The listing builds one solid part. Answer for the finished solid, in the listing's coordinates (mm). Face numbers are marked on the shaded views. A direction names the side the tool comes from. Give positions to 0.01 mm unless a question says otherwise; leave off trailing zeros. Order: outer loops, then holes, each group sorted by start corner. A loop starts at its lowest first (then second) coordinate and runs counter-clockwise, first axis right, second up. Notation, with made-up numbers: (-22.75, 14.25) -> (18.25, 14.25) arc R29 cw to (18.25, 49.25) -> close; hole circle Ø5 at (-2.5, 35.25). An arc over 180 degrees is marked (long way). Answer as a JSON object with one key per item and string values. Group by question number.
Autodesk Inventor part; units mm, degrees
ref_plane "YZ Plane" through (0, 0, 0) normal (1, 0, 0) x (0, 1, 0)
ref_plane "XZ Plane" through (0, 0, 0) normal (0, 1, 0) x (-1, 0, 0)
ref_plane "XY Plane" through (0, 0, 0) normal (0, 0, 1) x (1, 0, 0)
sketch "Sketch1" plane through (0, 0, 0) normal (0, 1, 0) x (-1, 0, 0)
  line L0 (22.5, 35) -> (-22.5, 35)
  line L1 (-22.5, 35) -> (-22.5, -35)
  line L2 (-22.5, -35) -> (22.5, -35)
  line L3 (22.5, -35) -> (22.5, 35)
  line L4 (22.5, 35) -> (-22.5, -35) construction
  line L5 (-22.5, 35) -> (22.5, -35) construction
  line L6 (0, 0) -> (0, -35) construction
  circle A0 centre (0, -25) radius 2.5
  circle A1 centre (0, -25) radius 4.5 construction
  line L7 (0, -25) -> (-4.5, -25) construction
  circle A2 centre (-4.5, -25) radius 0.625
  circle A3 centre (-6.5, -25) radius 0.625
  circle A4 centre (-8.5, -25) radius 0.625
  circle A5 centre (-10.5, -25) radius 0.625
  circle A6 centre (-12.5, -25) radius 0.625
  circle A7 centre (-14.5, -25) radius 0.625
  circle A8 centre (4.5, -25) radius 0.625
  circle A9 centre (6.5, -25) radius 0.625
  circle A10 centre (8.5, -25) radius 0.625
  circle A11 centre (10.5, -25) radius 0.625
  circle A12 centre (12.5, -25) radius 0.625
  circle A13 centre (14.5, -25) radius 0.625
  dimension "d3" = 9
  dimension "d0" = 45
  dimension "d1" = 70
  dimension "d2" = 5
  dimension "d4" = 1.25
  dimension "d7" = 2
  dimension "d14" = 360
  dimension "d16" = 10
extrude "Extrusion1" add sketch "Sketch1" along normal blind 3.175
fillet "Fillet1" radius 3.175 4 edges at (22.5, 1.5875, -35) (-22.5, 1.5875, -35) (-22.5, 1.5875, 35) (22.5, 1.5875, 35)
sketch "Sketch2" plane through (0, 3.175, 0) normal (0, 1, 0) x (1, 0, 0)
  line L0 (-22.5, 31.825) -> (-22.5, -31.825)
  line L1 (-22.5, 15) -> (22.5, 15)
  line L2 (22.5, -31.825) -> (22.5, 31.825)
  line L3 (19.325, 35) -> (-19.325, 35)
  point P0 (0, 0)
  dimension "d20" = 20
bend part "Bend Part1" radius 3 angle 90 line through (-22.5, 3.175, -15) along (1, 0, 0) centre toward (0, 1, 0) moving side (0, 0, -1) both sides no
properties part number "Platform"
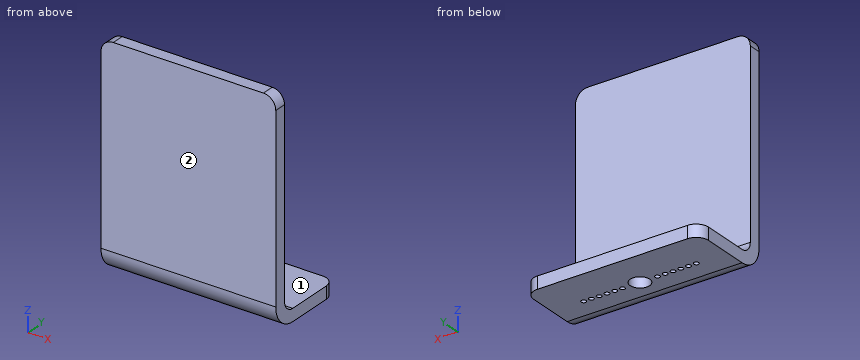
(1) A cutting plane is placed at A-A (x = 0). Determine the outline of the cut face in (y, z) (3 decimals).
(2) A cutting plane is placed at C-C (y = 17.25). Determine the outline of the cut face in (x, z) (3 decimals).
(3) A cutting plane is placed at D-D (z = 12). Determine the outline of the cut face in (x, y) (3 decimals).
(4) Find the intervals of material crossed by line 1 along Y through (x, z) = (-2, 33) (3 decimals); line 2 along Z through (x, y) = (-3.5, 17) (3 decimals); line 3 along Y through (x, z) = (10.5, -20.3), in increasing order. Write a range as [from, to].
(5) Which of the six approach directions +Z, -Z, +X, -X, +Y, -Y give full straight-line access (tool end or side, diameter ignored) to the marked faces 1 and 2?
(6) Flat-ended cylindrical pins translate along their axes: pin 1 Ø2 at (x, y) = (6.5, 11.46) entering from -Z (3 decimals); pin 2 Ø2 at (x, z) = (-9, 11) entering from +Y (3 decimals); pin 3 Ø12 at (x, y) = (-10, 16) entering from +Z. Find the tip coordinate at first contact, or state that the pin passes through.
(7) A cutting plane is placed at B-B (x = -10.5). Determine the outline of the cut face in (y, z) (3 decimals).
Check sheet entries:
{
 "1": {"outline": "(0, -15) arc R6.175 ccw to (6.175, -21.175) -> (8.963, -21.175) -> (8.963, -18) -> (6.175, -18) arc R3 cw to (3.175, -15) -> (3.175, 35) -> (0, 35) -> close; (13.963, -21.175) -> (21.463, -21.175) -> (21.463, -18) -> (13.963, -18) -> close"},
 "2": {"outline": "(-22.5, -21.175) -> (22.5, -21.175) -> (22.5, -18) -> (-22.5, -18) -> close"},
 "3": {"outline": "(-22.5, 0) -> (22.5, 0) -> (22.5, 3.175) -> (-22.5, 3.175) -> close"},
 "4": {"line 1": "y = [0, 3.175]", "line 2": "z = [-21.175, -18]", "line 3": "y = [3.01, 10.84], [12.09, 21.46]"},
 "5": {"face 1": "+Z, +X, -X, +Y", "face 2": "+Z, -Z, +X, -X, -Y"},
 "6": {"pin 1": "stops at z = -21.175", "pin 2": "stops at y = 3.175", "pin 3": "stops at z = -18"},
 "7": {"outline": "(0, -15) arc R6.175 ccw to (6.175, -21.175) -> (10.838, -21.175) -> (10.838, -18) -> (6.175, -18) arc R3 cw to (3.175, -15) -> (3.175, 35) -> (0, 35) -> close; (12.088, -21.175) -> (21.463, -21.175) -> (21.463, -18) -> (12.088, -18) -> close"}
}
